Autodesk Inventor part; units mm, degrees
ref_plane "Work Plane2" through (-255.2008, 77.7575, 0) normal (0, -1, 0) x (1, 0, 0)
ref_plane "YZ Plane" through (0, 0, 0) normal (1, 0, 0) x (0, 1, 0)
ref_plane "XZ Plane" through (0, 0, 0) normal (0, 1, 0) x (-1, 0, 0)
sketch "スケッチ2" plane through (0, 0, 0) normal (0, 0, 1) x (1, 0, 0)
  line L0 (-162.2425, 92.7575) -> (-162.2425, 62.7575)
  line L1 (-277.2425, 207.7575) -> (-237.2425, 207.7575)
  arc A0 (-290.563, 75.2382) -> (-273.922, 50.2767) centre (-282.2425, 62.7575) ccw
  line L2 (-277.2425, 84.1186) -> (-290.563, 75.2382)
  line L3 (-277.2425, 84.1186) -> (-277.2425, 207.7575)
  line L4 (-237.2425, 207.7575) -> (-237.2425, 92.7575)
  line L5 (-237.2425, 92.7575) -> (-162.2425, 92.7575)
  line L6 (-273.922, 50.2767) -> (-255.2008, 62.7575)
  line L7 (-255.2008, 62.7575) -> (-162.2425, 62.7575)
  line L8 (-282.2425, 62.7575) -> (-237.2425, 92.7575) construction
  point P0 (0, 0)
  dimension "d18" = 120
  dimension "d21" = 15
  dimension "d116" = 5
  dimension "d154" = 15
  dimension "d155" = 145
  dimension "d175" = 30
  dimension "d181" = 90
  dimension "d182" = 40
extrude "押し出し2" add sketch "スケッチ2" along normal blind 12
sketch "スケッチ3" plane through (0, 0, 12) normal (0, 0, 1) x (1, 0, 0)
  arc A0 (-290.563, 75.2382) -> (-282.2425, 47.7575) centre (-282.2425, 62.7575) ccw
  line L0 (-267.2425, 207.7575) -> (-237.2425, 207.7575)
  point P0 (-257.2425, 185.2575)
  dimension "d16" = 25
  dimension "d153" = 22.5
hole "穴1" at (-257.2425, 185.2575, 12) at (-282.2425, 62.7575, 12) direction (0, 0, -1) diameter 14 end through all
sketch "スケッチ10" plane through (-237.2425, 92.7575, 0) normal (0, 1, 0) x (1, 0, 0)
  line L0 (75, 0) -> (75, -12)
  line L1 (0, -12) -> (75, -12)
  line L2 (75, 0) -> (0, 0)
  point P0 (65, -6)
  point P1 (30, -6)
  dimension "d119" = 35
  dimension "d156" = 10
  dimension "d157" = 6
hole "穴8" at (-172.2425, 92.7575, 6) at (-207.2425, 92.7575, 6) direction (0, -1, 0) diameter 6.6 end through all
chamfer "面取り1" distance 5 angle 45 1 edges at (-162.2425, 62.7575, 6)
fillet "フィレット1" radius 10 1 edges at (-237.2425, 92.7575, 6)
chamfer "面取り2" distance 5 angle 45 1 edges at (-237.2425, 207.7575, 6)
ref_plane "Work Plane2" through (-255.2008, 77.7575, 0) normal (0, -1, 0) x (1, 0, 0)
sketch "Sketch18" plane through (0, 0, 0) normal (0, 0, -1) x (-1, 0, 0)
  line L0 (162.2425, 67.7575) -> (162.2425, 92.7575)
  line L1 (324.2425, 77.7575) -> (135.2425, 77.7575) construction
  point P0 (187.2425, 77.7575)
  dimension "d165" = 25
hole "Hole13" at (-187.2425, 77.7575, 0) direction (0, 0, 1) diameter 9 end through all
pattern_linear "Rectangular Pattern1" count 2 spacing 35 along (-1, 0, 0) of "Hole13"
fillet "Fillet2" radius 15 2 edges at (-255.2008, 62.7575, 6) (-277.2425, 84.1186, 6)
chamfer "Chamfer3" distance 10 angle 45 1 edges at (-277.2425, 207.7575, 6)
properties part number "Support Bracket" material "STEEL - MILD"
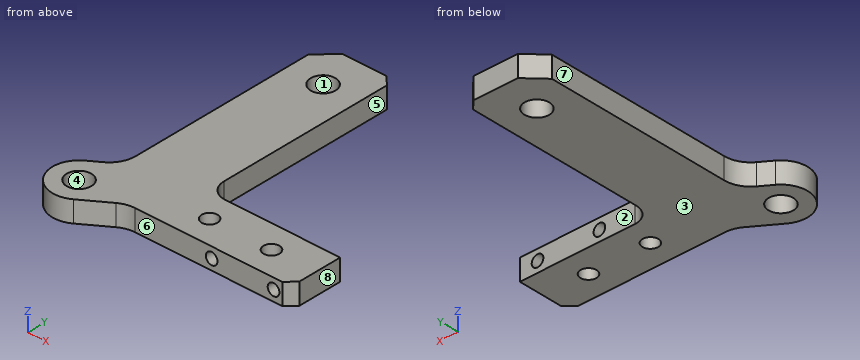
Check sheet for the modelled part. Datum: model origin and axes. Units: mm. Face numbers are marked on the shaded views. A direction names the side the tool comes from. Round coordinates to 2 decimals unless told otherwise and drop trailing zeros. Order: outer loops, then holes, each group sorted by start corner. A loop starts at its lowest first (then second) coordinate and runs counter-clockwise, first axis right, second up. Notation, with made-up numbers: (22, 65.5) -> (59, 65.5) arc R21 ccw to (59, 96.5) -> close; hole circle Ø11 at (86.5, -5.5). An arc over 180 degrees is marked (long way). One line per item, written item: value. Start each with the question number.
Q1. Mould release check, pull along Y, two halves, no side actions. Record for the marked faces 1, 2, 3 and 4: pulls with the +Y half, pulls with the -Y half, needs draft (parallel to the pull), parting line crosses it, or undercut.
Q2. Cross-section at B-B (x = -262). Record the boundary of the cut face in (y, z), and give its area (3 significant figures).
Q3. Cross-section at D-D (x = -216). Record the boundary of the cut face in (y, z), and give its area (3 significant figures).
Q4. Gauge pin test, flat ends, axial feed: pin 1 Ø6 at (y, z) = (140.5, 3.5) entering from -X; pin 2 Ø1 at (x, z) = (-238.5, 4.5) entering from +Y (3 decimals); pin 3 Ø8 at (x, y) = (-222.24, 77.76) entering from -Z; pin 4 Ø4 at (x, z) = (-236.5, 10) entering from +Y (3 decimals). Record the tip position at first contact, or that the pin passes through.
Q5. Set-up check for the marked faces 5, 6, 7 and 8: record each of +Z, -Z, +X, -X, +Y, -Y from which the full face is reachable in a straight line by a thin tool's end or side.
Q6. Cross-section at A-A (z = 7). Record the boundary of the cut face in (x, y), and give its area (3 significant figures).
Q7. Cross-section at C-C (y = 123). Record the boundary of the cut face in (x, z).
Q8. Thickness scan on line 1 (Y direction, x = -222, z = 1.25); line 2 (X direction, y = 66, z = 8.25); line 3 (X direction, y = 152, z = 10.75). Record the ranges inside material, lowest first.
Completed:
1. face 1: undercut
1. face 2: pulls with the +Y half
1. face 3: needs draft
1. face 4: undercut
2. outline: (58.22, 0) -> (180.12, 0) -> (180.12, 12) -> (58.22, 12) -> close; (190.39, 0) -> (207.76, 0) -> (207.76, 12) -> (190.39, 12) -> close
2. area: 1,670 mm²
3. outline: (62.76, 0) -> (92.76, 0) -> (92.76, 12) -> (62.76, 12) -> close
3. area: 360 mm²
4. pin 1: stops at x = -277.24
4. pin 2: stops at y = 204.515
4. pin 3: passes through
4. pin 4: stops at y = 204.015
5. face 5: +Z, -Z, +X, +Y
5. face 6: +Z, -Z, +X, -Y
5. face 7: +Z, -Z, -X, +Y
5. face 8: +Z, -Z, +X, +Y, -Y
6. outline: (-290.56, 75.24) arc R15 ccw to (-273.92, 50.28) -> (-258.98, 60.24) arc R15 cw to (-250.66, 62.76) -> (-210.39, 62.76) -> (-210.39, 92.76) -> (-227.24, 92.76) arc R10 cw to (-237.24, 102.76) -> (-237.24, 202.76) -> (-242.24, 207.76) -> (-267.24, 207.76) -> (-277.24, 197.76) -> (-277.24, 92.15) arc R15 cw to (-283.92, 79.67) -> close; (-204.1, 62.76) -> (-175.39, 62.76) -> (-175.39, 92.76) -> (-204.1, 92.76) -> close; (-169.1, 62.76) -> (-167.24, 62.76) -> (-162.24, 67.76) -> (-162.24, 92.76) -> (-169.1, 92.76) -> close; hole circle Ø14 at (-282.24, 62.76); hole circle Ø14 at (-257.24, 185.26); hole circle Ø9 at (-222.24, 77.76); hole circle Ø9 at (-187.24, 77.76)
6. area: 7,890 mm²
7. outline: (-277.24, 0) -> (-237.24, 0) -> (-237.24, 12) -> (-277.24, 12) -> close
8. line 1: y = 62.76 to 73.26, 82.25 to 92.76
8. line 2: x = -296.89 to -288.45, -276.04 to -209.66, -204.83 to -174.66, -169.83 to -164
8. line 3: x = -277.24 to -237.24
